```python
from build123d import *

# Parameters (mm, degrees)
BOSS_EXTRUDE1_DEPTH = 5


with BuildPart() as part:
    # Sketch1 → Boss-Extrude1 (new body)
    with BuildSketch(Plane(origin=(0, 0, 0), x_dir=(1, 0, 0), z_dir=(0, 1, 0))):
        with BuildLine():
            Line((-65.607722973, 30.584051311), (-58.536655161, 37.655119123))
            Line((-58.536655161, 37.655119123), (-45.801042376, 24.919506337))
            ThreePointArc((-45.801042376, 24.919506337), (-44.557414065, 23.404140856), (-43.633314863, 21.675272849))
            Line((-43.633314863, 21.675272849), (-41.465587349, 16.441915687))
            Line((-41.465587349, 16.441915687), (-31.465587349, 16.441915687))
            Line((-31.465587349, 16.441915687), (-28.536655161, 23.512983499))
            Line((-28.536655161, 23.512983499), (-14.394519538, 37.655119123))
            Line((-14.394519538, 37.655119123), (-7.323451726, 30.584051311))
            Line((-7.323451726, 30.584051311), (-18.536655161, 19.370847875))
            ThreePointArc((-18.536655161, 19.370847875), (-20.704382675, 16.126614387), (-21.465587349, 12.299780063))
            Line((-21.465587349, 12.299780063), (-21.465587349, -29.415948689))
            ThreePointArc((-21.465587349, -29.415948689), (-20.704382675, -33.242783013), (-18.536655161, -36.487016501))
            Line((-18.536655161, -36.487016501), (-7.323451726, -47.700219937))
            Line((-7.323451726, -47.700219937), (-14.394519538, -54.771287748))
            Line((-14.394519538, -54.771287748), (-27.130132323, -42.035674963))
            ThreePointArc((-27.130132323, -42.035674963), (-28.373760634, -40.520309481), (-29.297859836, -38.791441475))
            Line((-29.297859836, -38.791441475), (-31.465587349, -33.558084313))
            Line((-31.465587349, -33.558084313), (-41.465587349, -33.558084313))
            Line((-41.465587349, -33.558084313), (-43.633314863, -38.791441475))
            ThreePointArc((-43.633314863, -38.791441475), (-44.557414065, -40.520309481), (-45.801042376, -42.035674963))
            Line((-45.801042376, -42.035674963), (-58.536655161, -54.771287748))
            Line((-58.536655161, -54.771287748), (-65.607722973, -47.700219937))
            Line((-65.607722973, -47.700219937), (-54.394519538, -36.487016501))
            ThreePointArc((-54.394519538, -36.487016501), (-52.226792024, -33.242783013), (-51.465587349, -29.415948689))
            Line((-51.465587349, -29.415948689), (-51.465587349, 12.299780063))
            ThreePointArc((-51.465587349, 12.299780063), (-52.226792024, 16.126614387), (-54.394519538, 19.370847875))
            Line((-54.394519538, 19.370847875), (-65.607722973, 30.584051311))
        make_face()
    extrude(amount=BOSS_EXTRUDE1_DEPTH)


solid = part.part
```
Input: part model. Units: mm. Frame: model coordinates. A direction names the side the tool comes from. Coordinates: 2 decimals unless noted, no trailing zeros. Write each loop counter-clockwise with the first axis right and the second up, starting at its lowest first coordinate (ties: lowest second). Pieces come first, ordered by that corner, then holes.
1) Section A-A on x = -12.5. Output: boundary loops of the cut face in (y, z).
2) Material intervals for line 1 along X through (y, z) = (1.25, -11); line 2 along Z through (x, y) = (-31.5, 1.05); line 3 along X through (y, z) = (2.25, -24), sorted ascending.
3) Set-up query: faces 4 (the flat face through (-60.08, 2.46, 42.17)), 5 (the flat face through (-42.534, 2.465, 36.138)), 6 (the flat face through (-30.02, 2.46, -19.93)). Return all of +Z, -Z, +X, -X, +Y, -Y with unobstructed straight access to the full face (end or side cutting, diameter ignored); none if empty.
4) Pin query (flat end, axial travel): pin 1 Ø3 at (y, z) = (1, 10.5) entering from +X; pin 2 Ø2.5 at (y, z) = (1.5, 6) entering from -X; pin 3 Ø3 at (x, y) = (-18, 2.5) entering from +Z. Return the tip coordinate at first contact, or that it passes through.
5) Section D-D on z = 17. Output: boundary loops of the cut face in (x, y).
6) Mould query, pull axis Z, two halves, no side actions, for faces 1 (the flat face through (-21.56, 2.46, -30.49)), 2 (the flat face through (-36, 5, 8)), 3 (the cylindrical face through (-52.248, 2.465, 33.294)). Classes: pulls with the +Z half, pulls with the -Z half, needs draft (parallel to the pull), parting line crosses it, or undercut.
7) Section C-C on z = 44.5. Output: boundary loops of the cut face in (x, y), and give its area (3 significant figures).
8) Section B-B on y = 3.7. Output: boundary loops of the cut face in (x, z).
Check result:
1. outline: (0, -35.76) - (5, -35.76) - (5, -25.41) - (0, -25.41) - close; (0, 42.52) - (5, 42.52) - (5, 52.88) - (0, 52.88) - close
2. line 1: x = -51.47 to -21.47
2. line 2: z = -16.44 to 33.56
2. line 3: x = -59.02 to -44.99, -28.05 to -13.91
3. face 4: -X, +Y, -Y
3. face 5: +Z, +Y, -Y
3. face 6: -Z, +Y, -Y
4. pin 1: stops at x = -21.47
4. pin 2: stops at x = -51.47
4. pin 3: stops at z = 52.67
5. outline: (-51.47, 0) - (-21.47, 0) - (-21.47, 5) - (-51.47, 5) - close
6. face 1: pulls with the -Z half
6. face 2: needs draft
6. face 3: undercut
7. outline: (-62.41, 0) - (-48.27, 0) - (-48.27, 5) - (-62.41, 5) - close; (-24.67, 0) - (-10.52, 0) - (-10.52, 5) - (-24.67, 5) - close
7. area: 141 mm2
8. outline: (-65.61, -30.58) - (-58.54, -37.66) - (-45.8, -24.92) arc R10 ccw to (-43.63, -21.68) - (-41.47, -16.44) - (-31.47, -16.44) - (-28.54, -23.51) - (-14.39, -37.66) - (-7.32, -30.58) - (-18.54, -19.37) arc R10 cw to (-21.47, -12.3) - (-21.47, 29.42) arc R10 cw to (-18.54, 36.49) - (-7.32, 47.7) - (-14.39, 54.77) - (-27.13, 42.04) arc R10 ccw to (-29.3, 38.79) - (-31.47, 33.56) - (-41.47, 33.56) - (-43.63, 38.79) arc R10 ccw to (-45.8, 42.04) - (-58.54, 54.77) - (-65.61, 47.7) - (-54.39, 36.49) arc R10 cw to (-51.47, 29.42) - (-51.47, -12.3) arc R10 cw to (-54.39, -19.37) - close
